```python
from build123d import *
from OCP.BRepFilletAPI import BRepFilletAPI_MakeChamfer

# Parameters (mm, degrees)
SKETCH9_R           = 2
BOSS_EXTRUDE3_DEPTH = 14
SKETCH10_R          = 2
CUT_EXTRUDE7_DEPTH  = 14
SKETCH11_W          = 9
SKETCH11_H          = 26.686138344
CUT_EXTRUDE8_DEPTH  = 28
FILLET1_R           = 2
CHAMFER1_SIZE       = 2.5
CHAMFER1_SIZE2      = 4.365846821
CHAMFER1_SIZE2_2    = 4.330127019
EXTRUDE1_DEPTH      = 3
EXTRUDE1_DEPTH_BACK = 3
FILLET2_R           = 4


with BuildPart() as part:
    # Sketch9 → Boss-Extrude3 (new body)
    with BuildSketch(Plane(origin=(0, 0, 0), x_dir=(0, 0, -1), z_dir=(1, 0, 0))):
        with BuildLine():
            Line((8, 5.053889445), (8, -49.642014822))
            Line((8, -49.642014822), (-8, -49.642014822))
            Line((-8, -49.642014822), (-8, -10.875806049))
            ThreePointArc((-8, -10.875806049), (-8.427714838, -7.982476346), (-9.674271354, -5.336650652))
            ThreePointArc((-9.674271354, -5.336650652), (-7.418447874, 8.870328147), (6.925281884, 7.78202542))
            ThreePointArc((6.925281884, 7.78202542), (7.721634556, 6.519985019), (8, 5.053889445))
        make_face()
        Circle(SKETCH9_R, mode=Mode.SUBTRACT)
        with BuildLine():
            Line((5.5, -41.5), (5.5, -25.762364524))
            ThreePointArc((5.5, -25.762364524), (3.987567872, -22.111030369), (0.336233717, -20.598598241))
            Line((0.336233717, -20.598598241), (-0.410415455, -20.598598241))
            ThreePointArc((-0.410415455, -20.598598241), (-4.070351606, -22.119652678), (-5.574124284, -25.786723302))
            Line((-5.574124284, -25.786723302), (-5.5, -41.5))
            Line((-5.5, -41.5), (5.5, -41.5))
        make_face(mode=Mode.SUBTRACT)
    extrude(amount=BOSS_EXTRUDE3_DEPTH)

    # Sketch10 → Cut-Extrude7 (cut)
    with BuildSketch(Plane.XZ.offset(49.642014822)):
        with Locations(Location((7, 0, 0), (0, 0, 270))):
            Circle(SKETCH10_R)
    extrude(amount=-CUT_EXTRUDE7_DEPTH, mode=Mode.SUBTRACT)

    # Sketch11 → Cut-Extrude8 (cut)
    with BuildSketch(Plane(origin=(0, 16, 0), x_dir=(1, 0, 0), z_dir=(0, 1, 0))):
        with Locations((7, -2.737831409)):
            Rectangle(SKETCH11_W, SKETCH11_H)
    extrude(amount=-CUT_EXTRUDE8_DEPTH, mode=Mode.SUBTRACT)

    # Fillet1
    fillet1_edges = [part.edges().sort_by_distance(p)[0] for p in [
        (7, -49.642014822, 8),
        (7, -49.642014822, -8),
    ]]
    fillet(fillet1_edges, radius=FILLET1_R)

    # Chamfer1: one chamfer whose edges measure the first distance from different faces: ONE call of the kernel's chamfer builder (chamfer() names one face for all edges)
    chamfer1_edges_1 = [part.edges().sort_by_distance(p)[0] for p in [
        (7, -41.5, 5.5),
    ]]
    chamfer1_side_1 = [part.faces().sort_by_distance(p)[0] for p in [
        (7, -41.5, 5.321955062),
    ]]
    chamfer1_edges_2 = [part.edges().sort_by_distance(p)[0] for p in [
        (7, -41.5, -5.5),
    ]]
    chamfer1_side_2 = [part.faces().sort_by_distance(p)[0] for p in [
        (7, -41.5, 5.321955062),
    ]]
    chamfer1 = BRepFilletAPI_MakeChamfer(part.part.solid().wrapped)
    for e in chamfer1_edges_1:
        chamfer1.Add(CHAMFER1_SIZE, CHAMFER1_SIZE2, e.wrapped, chamfer1_side_1[0].wrapped)  # the first distance lies on this face
    for e in chamfer1_edges_2:
        chamfer1.Add(CHAMFER1_SIZE, CHAMFER1_SIZE2_2, e.wrapped, chamfer1_side_2[0].wrapped)  # the first distance lies on this face
    add(Compound.cast(chamfer1.Shape()), mode=Mode.REPLACE)

    # Sketch12 → Extrude1 (cut, two sides)
    with BuildSketch(Plane(origin=(0, -41.5, 0), x_dir=(1, 0, 0), z_dir=(0, 1, 0))) as extrude1_sk:
        Polygon((7, 4.3), (3.276090764, 2.15), (3.276090764, -2.15), (7, -4.3), (10.723909236, -2.15), (10.723909236, 2.15), align=None)
    extrude(amount=EXTRUDE1_DEPTH, mode=Mode.SUBTRACT)
    extrude(extrude1_sk.sketch, amount=-EXTRUDE1_DEPTH_BACK, mode=Mode.SUBTRACT)

    # Fillet2
    fillet2_edges = [part.edges().sort_by_distance(p)[0] for p in [
        (2.5, -12, 0),
        (11.5, -12, 0),
    ]]
    fillet(fillet2_edges, radius=FILLET2_R)


solid = part.part
```
Work out the finished part from the listing and answer in its coordinate system (mm). A direction names the side the tool comes from. Give positions to 0.01 mm unless a question says otherwise; leave off trailing zeros. Write each loop counter-clockwise with the first axis right and the second up, starting at its lowest first coordinate (ties: lowest second). Pieces come first, ordered by that corner, then holes. Notation, with made-up numbers: (-22, 38) -> (30, 38) arc R6 ccw to (30, 49) -> close; hole circle Ø5 at (-20, 7.5). An arc over 180 degrees is marked (long way). Write item = value, one per line.
Q1. For a pull along Z with two mould halves and no side action, classify faces 6 (the flat face through (7, -32, -5.5)), 7 (the cylindrical face through (1.23, 8.73, 7.59)), 8 (the flat face through (7, -30, 8)), 9 (the flat face through (5.58, -42.42, -3.48)) as pulls with the +Z half, pulls with the -Z half, needs draft (parallel to the pull), parting line crosses it, or undercut.
Computed values:
face_6 = undercut
face_7 = parting line crosses it
face_8 = pulls with the +Z half
face_9 = undercut
Q2. Consider line 1 along X through (y, z) = (3, -6.75); line 2 along Y through (x, z) = (12.9, 0); line 3 along Z through (x, y) = (4.75, -41.5). Determine where each line is inside the solid, lowest interval first.
Computed values:
line_1 = 0 to 2.5, 11.5 to 14
line_2 = -49.64 to -41.5, -20.6 to -2, 2 to 11.12
line_3 = -8 to -3, 3 to 8
Q3. Section D-D on y = 0 is taken. Determine the outline of the cut face in (x, z).
Computed values:
outline = (0, -8) -> (2.5, -8) -> (2.5, -2) -> (0, -2) -> close; (0, 2) -> (2.5, 2) -> (2.5, 11.44) -> (0, 11.44) -> close; (11.5, -8) -> (14, -8) -> (14, -2) -> (11.5, -2) -> close; (11.5, 2) -> (14, 2) -> (14, 11.44) -> (11.5, 11.44) -> close
Q4. Section C-C on y = -28 is taken. Determine the outline of the cut face in (x, z), and give its area (3 significant figures).
Computed values:
outline = (0, -8) -> (14, -8) -> (14, -5.5) -> (0, -5.5) -> close; (0, 5.56) -> (14, 5.56) -> (14, 8) -> (0, 8) -> close
area = 69.1 mm^2
Q5. Flat-ended cylindrical pins translate along their axes: pin 1 Ø3.5 at (x, z) = (7, 0) entering from +Y; pin 2 Ø6 at (x, y) = (10.5, -16.5) entering from +Z; pin 3 Ø3.5 at (x, z) = (6.5, -2) entering from +Y; pin 4 Ø6 at (x, y) = (10, 4) entering from -Z. Find the tip coordinate at first contact, or state that the pin passes through.
Computed values:
pin_1 = -11.8
pin_2 = 8
pin_3 = -11.6
pin_4 = -8
Q6. Section B-B on y = -43.5 is taken. Determine the outline of the cut face in (x, z).
Computed values:
outline = (0, -8) -> (14, -8) -> (14, 8) -> (0, 8) -> close; hole (3.28, -2.15) -> (7, -4.3) -> (10.72, -2.15) -> (10.72, 2.15) -> (7, 4.3) -> (3.28, 2.15) -> close
Q7. A tool of negligible diameter and unlimited length cuts with its end or side. For faces 1 (the cylindrical face through (1.232, 6.54, -7.714)), 2 (the flat face through (8.47, -42.49, -3.45)), 3 (the flat face through (6.902, -38.824, -4.545)), 4 (the cylindrical face through (3.641, -10.797, 0.096)), 5 (the flat face through (14, -12, -1)), from which of +Z, -Z, +X, -X, +Y, -Y can it reach the whole face along a straight path? Write none if from no direction.
Computed values:
face_1 = -Z, +X, -X, +Y
face_2 = none
face_3 = +X, -X
face_4 = +Z, -Z, +Y
face_5 = +Z, -Z, +X, +Y, -Y
Q8. Section A-A on x = 12.5 is taken. Determine the outline of the cut face in (y, z).
Computed values:
outline = (-49.64, -6) arc R2 ccw to (-47.64, -8) -> (5.05, -8) arc R4 ccw to (7.78, -6.93) arc R10.61 ccw to (-5.34, 9.67) arc R10 cw to (-10.88, 8) -> (-47.64, 8) arc R2 ccw to (-49.64, 6) -> close; hole (-41.5, -3) -> (-37.17, -5.5) -> (-25.76, -5.5) arc R5.16 ccw to (-20.6, -0.34) -> (-20.6, 0.41) arc R5.16 ccw to (-25.79, 5.57) -> (-37.13, 5.52) -> (-41.5, 3) -> close; hole circle Ø4 at (0, 0)
